Can you work these out from the model? Positions are in its coordinate system, mm. A direction names the side the tool comes from. Round coordinates to 2 decimals unless told otherwise and drop trailing zeros. Write each loop counter-clockwise with the first axis right and the second up, starting at its lowest first coordinate (ties: lowest second). Pieces come first, ordered by that corner, then holes. Notation, with made-up numbers: M 34.5,71 L 63.5,71 A30 ccw 63.5,96 Z; hole C 56,77 d11. An arc over 180 degrees is marked long. Answer in a Markdown table with one row per item. Add a question column.
(1) If we mould it in two halves opening along Y, with no side actions, what happens to faces 1 (the face through (16.82, 0.03, -0.01)), 2 (the face through (-2, 0, -3)), 3 (the face through (6.69, -0.03, -1.34))? For each: released by +Y, released by -Y, zero draft, split by the parting line, or undercut.
(2) Suppose I cut it at B-B, the plane z = 0.6. Write out the boundary of the cut face in (x, y), then the cut area to 3 significant figures.
(3) Suppose I cut it at D-D, the plane x = 9. Write out the boundary of the cut face in (y, z).
(4) For faces 4 (the face through (1, 0, -1.95)), 5 (the face through (14, 0, -0.85)), 6 (the face through (9, 2, 0)), which set-ups out of +Z, -Z, +X, -X, +Y, -Y let a thin tool reach every point of the face, with its end or its side?
(5) I'm going to push flat-ended pins straight in: pin 1 (2 mm diameter, centred on y = 0, z = -1, fed in from -X); pin 2 (1 mm diameter, centred on y = 0, z = -3, fed in from +X); pin 3 (0.6 mm diameter, centred on y = 1, z = -0.5, fed in from -X). Where does each tip first touch, or does it pass through?
(6) Suppose I cut it at C-C, the plane y = 0. Count the separate pieces of the cut face and the enclosed holes in it, then the cut area to 3 significant figures.
(7) If I drill on probe 1 along Y at (x, z) = (0, -2.9); probe 2 along Z at (x, y) = (17.25, 1.35); probe 3 along X at (y, z) = (-0.45, -0.4), over which ranges is the centre line in solid material (lowest first)?
(8) Suppose I cut it at A-A, the plane x = 0.5. Write out the boundary of the cut face in (y, z), then the cut area to 3 significant figures.
from build123d import *

# Parameters (mm, degrees)
SKETCH1_R           = 0.75
BOSS_EXTRUDE1_DEPTH = 0.85
SKETCH2_R           = 0.75
BOSS_EXTRUDE2_DEPTH = 2.5
SKETCH3_R           = 0.75
CUT_EXTRUDE1_DEPTH  = 2.8
FILLET1_R           = 2
FILLET2_R           = 1
FILLET3_R           = 1


with BuildPart() as part:
    # Sketch1 → Boss-Extrude1 (new body, symmetric)
    with BuildSketch(Plane.XY):
        with BuildLine():
            Line((0, 2), (17.57, 2))
            ThreePointArc((17.57, 2), (19.57, 0), (17.57, -2))
            Line((17.57, -2), (0, -2))
            ThreePointArc((0, -2), (-2, 0), (0, 2))
        make_face()
        Circle(SKETCH1_R, mode=Mode.SUBTRACT)
        with Locations((17.57, 0)):
            Circle(SKETCH1_R, mode=Mode.SUBTRACT)
    extrude(amount=BOSS_EXTRUDE1_DEPTH, both=True)

    # Sketch2 → Boss-Extrude2 (add)
    with BuildSketch(Plane(origin=(0, 0, -0.85), x_dir=(-1, 0, 0), z_dir=(0, 0, -1))):
        with BuildLine():
            Line((-6, 2), (-6, -2))
            Line((-6, -2), (0, -2))
            ThreePointArc((0, -2), (2, 0), (0, 2))
            Line((0, 2), (-6, 2))
        make_face()
        Circle(SKETCH2_R, mode=Mode.SUBTRACT)
    extrude(amount=BOSS_EXTRUDE2_DEPTH)

    # Sketch3 → Cut-Extrude1 (cut)
    with BuildSketch(Plane.XY.offset(0.85)):
        with BuildLine():
            Line((4, 2), (4, -2))
            Line((4, -2), (0, -2))
            ThreePointArc((0, -2), (-2, 0), (0, 2))
            Line((0, 2), (4, 2))
        make_face()
        Circle(SKETCH3_R, mode=Mode.SUBTRACT)
    extrude(amount=-CUT_EXTRUDE1_DEPTH, mode=Mode.SUBTRACT)

    # Fillet1
    fillet1_edges = [part.edges().sort_by_distance(p)[0] for p in [
        (6, 0, -0.85),
    ]]
    fillet(fillet1_edges, radius=FILLET1_R)

    # Fillet2
    fillet2_edges = [part.edges().sort_by_distance(p)[0] for p in [
        (6, 0, -3.35),
    ]]
    fillet(fillet2_edges, radius=FILLET2_R)

    # Fillet3
    fillet3_edges = [part.edges().sort_by_distance(p)[0] for p in [
        (4, 0, -1.95),
        (4, 0, 0.85),
    ]]
    fillet(fillet3_edges, radius=FILLET3_R)


solid = part.part
Calculated:
| question | item | result |
|---|---|---|
| 1 | face 1 | undercut |
| 1 | face 2 | split by the parting line |
| 1 | face 3 | zero draft |
| 2 | outline | M 4.34,-2 L 17.57,-2 A2 ccw 17.57,2 L 4.34,2 Z; hole C 17.57,0 d1.5 |
| 2 | area | 57.4 mm² |
| 3 | outline | M -2,-0.85 L 2,-0.85 L 2,0.85 L -2,0.85 Z |
| 4 | face 4 | +Z, -X, +Y, -Y |
| 4 | face 5 | -Z, +X, +Y, -Y |
| 4 | face 6 | +Z, -Z, +X, -X, +Y |
| 5 | pin 1 | x = -2 |
| 5 | pin 2 | x = 6.03 |
| 5 | pin 3 | x = 4 |
| 6 | separate pieces | 3 |
| 6 | enclosed holes | 0 |
| 6 | area | 35.9 mm² |
| 7 | probe 1 | -2 to -0.75, 0.75 to 2 |
| 7 | probe 2 | -0.85 to 0.85 |
| 7 | probe 3 | 4 to 16.97, 18.17 to 19.52 |
| 8 | outline | M -2,-3.35 L -0.56,-3.35 L -0.56,-1.95 L -2,-1.95 Z; M 0.56,-3.35 L 2,-3.35 L 2,-1.95 L 0.56,-1.95 Z |
| 8 | area | 4.03 mm² |
